For this review, take the finished solid that the model builds, in its own axes (mm). A direction names the side the tool comes from. Give positions to 0.01 mm unless a question says otherwise; leave off trailing zeros. Order: outer loops, then holes, each group sorted by start corner. A loop starts at its lowest first (then second) coordinate and runs counter-clockwise, first axis right, second up. Notation, with made-up numbers: M 9,-27.5 L 49,-27.5 A23 ccw 49,0.5 Z; hole C -36,47.5 d10. An arc over 180 degrees is marked long. Use CSV: the item, a comma, the result in double quotes. Start each with the question number.
(1) Draft analysis for pull direction X (two halves, no side actions). For faces 3 (the face through (0, 10.654, 15)), 4 (the face through (-11.385, -3.105, 33.521)), 5 (the face through (2, -16, 21)), 6 (the face through (-26.217, -14.647, 17.745)), state which applies: pulls with the +X half, pulls with the -X half, needs draft (parallel to the pull), parting line crosses it, or undercut.
(2) Consider section A-A (x = 1). Write out the cut boundary in (y, z).
(3) Consider section C-C (z = 24). Write out the cut boundary in (x, y).
(4) Clearance check with flat-ended pins moving along their axes: P1, Ø5.5, axis at x = 13, y = 0, coming from the -Z side (3 decimals); P2, Ø10, axis at x = 7, y = 0, coming from the -Z side; P3, Ø8.5, axis at x = 13, y = 0, coming from the -Z side. State where each tip first meets the part, or that it passes through.
(5) Tool access review of faces 1 (the face through (27.5, 0, 17)), 2 (the face through (-10, 3, 32)): name each direction out of +Z, -Z, +X, -X, +Y, -Y from which nothing blocks a thin tool from reaching the whole face with its end or side.
(6) Consider section B-B (y = 0). Write out the cut boundary in (x, z), and give its area (3 significant figures).
(7) Consider section D-D (z = 14.5). Write out the cut boundary in (x, y), and give its area (3 significant figures).
(8) Wall thickness on L1, parallel to X at y = 0, z = 30.85; L2, parallel to Y at x = 13, z = 31; L3, parallel to X at y = 6, z = 7.5: over which ranges is each line inside the solid? List them lowest first. Write a range as from..to.
```python
from build123d import *

# Parameters (mm, degrees)
F0_W      = 55
F0_H      = 32
F1_DEPTH  = 35
F2_W      = 43.775738
F2_H      = 21.308826
F3_DEPTH  = 30
F4_R      = 4.5
F5_R      = 4.5
F6_DEPTH  = 10
F7_R      = 3.5
F8_DEPTH  = 3
F9_R      = 7
F10_DEPTH = 2


with BuildPart() as f1:
    # F0 (on Top) → F1 (new body)
    with BuildSketch(Plane.XY):
        Rectangle(F0_W, F0_H)
    extrude(amount=F1_DEPTH)

    # F2 (on Top) → F3 (cut)
    with BuildSketch(Plane.XY):
        Rectangle(F2_W, F2_H)
    extrude(amount=F3_DEPTH, mode=Mode.SUBTRACT)

    # F4
    f4_edges = [f1.edges().sort_by_distance(p)[0] for p in [
        (-27.5, -16, 17.5),
    ]]
    fillet(f4_edges, radius=F4_R)

    # F5 (on face) → F6 (cut)
    with BuildSketch(Plane.XZ.offset(16)):
        with Locations((1, 14.5)):
            Circle(F5_R)
    extrude(amount=-F6_DEPTH, mode=Mode.SUBTRACT)

    # F7 (on face) → F8 (cut)
    with BuildSketch(Plane.XY.offset(35)):
        with Locations((-13, 0)):
            Circle(F7_R)
        with Locations((13, 0)):
            Circle(F7_R)
    extrude(amount=-F8_DEPTH, mode=Mode.SUBTRACT)

    # F9 (on face) → F10 (cut)
    with BuildSketch(Plane(origin=(0, 0, 30), x_dir=(1, 0, 0), z_dir=(0, 0, -1))):
        with Locations((-13, 0)):
            Circle(F9_R)
        with Locations((13, 0)):
            Circle(F9_R)
    extrude(amount=-F10_DEPTH, mode=Mode.SUBTRACT)


solid = f1.part
```
Check result:
1,face 3,"undercut"
1,face 4,"undercut"
1,face 5,"needs draft"
1,face 6,"pulls with the -X half"
2,outline,"M -16,0 L -10.65,0 L -10.65,10 L -16,10 Z; M -16,19 L -10.65,19 L -10.65,30 L 10.65,30 L 10.65,0 L 16,0 L 16,35 L -16,35 Z"
3,outline,"M -27.5,-11.5 A4.5 ccw -23,-16 L 27.5,-16 L 27.5,16 L -27.5,16 Z; hole M -21.89,-10.65 L 21.89,-10.65 L 21.89,10.65 L -21.89,10.65 Z"
4,P1,"passes through"
4,P2,"stops at z = 30"
4,P3,"stops at z = 32"
5,face 1,"+Z, -Z, +X, +Y, -Y"
5,face 2,"-Z"
6,outline,"M -27.5,0 L -21.89,0 L -21.89,30 L -20,30 L -20,32 L -16.5,32 L -16.5,35 L -27.5,35 Z; M -9.5,32 L -6,32 L -6,30 L 6,30 L 6,32 L 9.5,32 L 9.5,35 L -9.5,35 Z; M 16.5,32 L 20,32 L 20,30 L 21.89,30 L 21.89,0 L 27.5,0 L 27.5,35 L 16.5,35 Z"
6,area,"514 mm^2"
7,outline,"M -27.5,-11.5 A4.5 ccw -23,-16 L -3.5,-16 L -3.5,-10.65 L -21.89,-10.65 L -21.89,10.65 L 21.89,10.65 L 21.89,-10.65 L 5.5,-10.65 L 5.5,-16 L 27.5,-16 L 27.5,16 L -27.5,16 Z"
7,area,"775 mm^2"
8,L1,"x = -27.5..-20, -6..6, 20..27.5"
8,L2,"y = -16..-7, 7..16"
8,L3,"x = -27.5..-21.89, 21.89..27.5"
